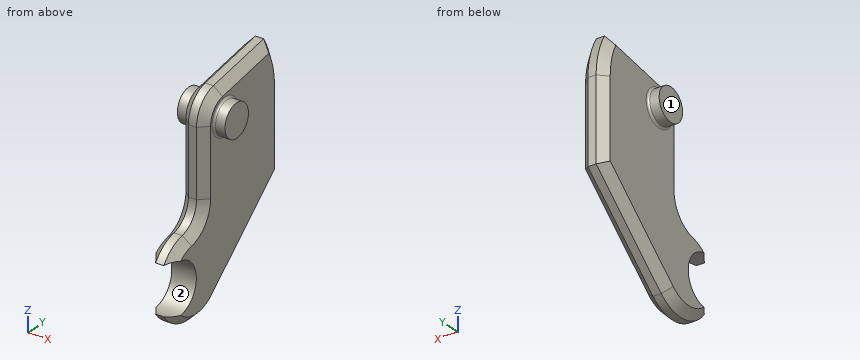
Autodesk Inventor part; units mm, degrees
ref_plane "YZ Plane" through (0, 0, 0) normal (1, 0, 0) x (0, 1, 0)
ref_plane "XZ Plane" through (0, 0, 0) normal (0, 1, 0) x (-1, 0, 0)
ref_plane "XY Plane" through (0, 0, 0) normal (0, 0, 1) x (1, 0, 0)
sketch "Sketch1" plane through (0, 0, 0) normal (1, 0, 0) x (0, 1, 0)
  arc A0 (9.4, 0) -> (7.9599, 5) centre (0, 0) ccw
  circle A1 centre (0, 0) radius 3.5
  line L0 (-0.6243, 3.4439) -> (7.9599, 5)
  line L1 (-3.5, 0) -> (-3.5, -8.9713)
  line L2 (9.4, 0) -> (9.4, -10)
  line L3 (-3.5, -8.9713) -> (-4.2585, -11.0553)
  line L4 (-3.5, -8.9713) -> (26.5, -8.9713) construction
  line L5 (-1.6991, -19.7555) -> (9.4, -10)
  arc A2 (-4.2585, -11.0553) -> (-1.6991, -19.7555) centre (-5, -16) ccw
  dimension "d0" = 18.8
  dimension "d2" = 7
  dimension "d4" = 5
  dimension "d5" = 10
  dimension "d7" = 110
  dimension "d26" = 10
  dimension "d27" = 5
  dimension "d28" = 16
extrude "Extrusion1" add sketch "Sketch1" along normal blind 3
sketch "Sketch2" plane through (3, 0, 0) normal (1, 0, 0) x (0, 0, -1)
  circle A0 centre (0, 0) radius 2
  dimension "d12" = 4
extrude "Extrusion2" add sketch "Sketch2" along normal blind 1.4
sketch "Sketch3" plane through (0, 0, 0) normal (-1, 0, 0) x (0, 0, 1)
  circle A0 centre (0, 0) radius 2
  dimension "d15" = 4
extrude "Extrusion3" add sketch "Sketch3" along normal blind 1.4
fillet "Fillet2" radius 3 2 edges at (1.5, -4.2585, -11.0553) (1.5, -3.5, -8.9713)
fillet "Fillet1" radius 0.25 2 edges at (3, 0, 2) (0, 0, -2)
chamfer "Chamfer2" distance 1 angle 45 14 edges at (0, 9.4, -5) (0, 9.0328, 2.6016) (3, 9.4, -5) (3, 9.0328, 2.6016) (0, 3.6678, 4.2219) (0, -2.6865, 2.2433) (0, -3.5, -4.0714) (0, -9.4918, -18.1964) (0, 3.8505, -14.8778) (3, 3.6678, 4.2219) (3, -2.6865, 2.2433) (3, -3.5, -4.0714) (3, -9.4918, -18.1964) (3, 3.8505, -14.8778)
sketch "Sketch5" plane through (3, 0, 0) normal (1, 0, 0) x (0, 0, -1)
  circle A0 centre (16, -8) radius 3.075
  point P0 (0, 0)
  dimension "d37" = 6.15
  dimension "d40" = 16
  dimension "d41" = 8
extrude "Extrusion5" cut sketch "Sketch5" against normal up to surface (3 mm away)
properties part number "TrainPullert"
For this review, take the finished solid that the model builds, in its own axes (mm). Face numbers are marked on the shaded views. Give positions to 0.01 mm unless a question says otherwise; leave off trailing zeros. Write each loop counter-clockwise with the first axis right and the second up, starting at its lowest first coordinate (ties: lowest second). Pieces come first, ordered by that corner, then holes. Notation, with made-up numbers: (30, 64.5) -> (81, 64.5) arc R21 ccw to (81, 82.5) -> close; hole circle Ø5 at (-29.5, 7). An arc over 180 degrees is marked (long way). Use CSV: the item, a comma, the result in double quotes.
Q1. Mouldability with a two-part tool opening along Z and no side actions: class the marked faces 1 and 2 as pulls with the +Z half, pulls with the -Z half, needs draft (parallel to the pull), parting line crosses it, or undercut.
Conclusion:
face 1,"needs draft"
face 2,"undercut"
Q2. For P1, Ø6, axis at y = -1.5, z = -17, coming from the +X side; P2, Ø1, axis at x = 2.5, y = -6, coming from the +Z side; P3, Ø0.8, axis at x = 1.5, z = -2.5, coming from the -Y side, all flat-tipped, find the tip position at first contact; note any pin that passes through.
Conclusion:
P1,"x = 3"
P2,"z = -11.09"
P3,"y = -3.5"
Q3. Take a section at B-B, the plane y = 0. Write out the cut boundary in (x, z).
Conclusion:
outline,"(-1.4, -2) -> (-0.25, -2) arc R0.25 cw to (0, -2.25) -> (0, -16.93) -> (1, -18.26) -> (2, -18.26) -> (3, -16.93) -> (3, -2.25) arc R0.25 cw to (3.25, -2) -> (4.4, -2) -> (4.4, 2) -> (3.25, 2) arc R0.25 cw to (3, 2.25) -> (3, 2.54) -> (2, 3.56) -> (1, 3.56) -> (0, 2.54) -> (0, 2.25) arc R0.25 cw to (-0.25, 2) -> (-1.4, 2) -> close"
Q4. Take a section at C-C, the plane x = -0.6. Write out the cut boundary in (y, z).
Conclusion:
outline,"circle Ø4 at (0, 0)"
Q5. Take a section at A-A, the plane z = -6.75. Write out the cut boundary in (x, y), then the cut area to 3 significant figures.
Conclusion:
outline,"(0, -2.5) -> (1, -3.5) -> (2, -3.5) -> (3, -2.5) -> (3, 8.4) -> (2, 9.4) -> (1, 9.4) -> (0, 8.4) -> close"
area,"36.7 mm2"
Q6. Take a section at D-D, the plane z = -14. Write out the cut boundary in (x, y), then the cut area to 3 significant figures.
Conclusion:
outline,"(0, -5.66) -> (3, -5.66) -> (3, 3.33) -> (2, 4.85) -> (1, 4.85) -> (0, 3.33) -> close"
area,"30.0 mm2"
Q7. To check wall thickness, follow probe 1 along X at (y, z) = (-2, -13.75); probe 2 along Z at (x, y) = (1.1, -8) (3 decimals); probe 3 along Z at (x, y) = (2.2, -8) (3 decimals). State the ranges of each line that lie inside material, in increasing order. Write a range as [from, to].
Conclusion:
probe 1,"[0, 3]"
probe 2,"[-20, -19.075], [-12.925, -12]"
probe 3,"[-19.747, -19.075], [-12.925, -12.253]"
